```python
from build123d import *

# Parameters (mm, degrees)
SKETCH1_R                    = 6.35
EXTRUDE1_DEPTH               = 22.225
F_5_16_18_TAPPED_HOLE1_D     = 6.5278
F_5_16_18_TAPPED_HOLE1_DEPTH = 20.32
F_5_16_18_TAPPED_HOLE1_TIP   = 1.961148974
F_5_16_18_TAPPED_HOLE2_D     = 6.5278
F_5_16_18_TAPPED_HOLE2_DEPTH = 20.32
F_5_16_18_TAPPED_HOLE2_TIP   = 1.961148974
SKETCH6_W                    = 0.9906
SKETCH6_H                    = 0.4064


with BuildPart() as part:
    # Sketch1 → Extrude1 (new body, symmetric)
    with BuildSketch(Plane.XY):
        Circle(SKETCH1_R)
    extrude(amount=EXTRUDE1_DEPTH, both=True)

    # 5/16-18 Tapped Hole1
    with Locations(Plane.XY.offset(22.225)):
        with Locations((0, 0)):
            Hole(F_5_16_18_TAPPED_HOLE1_D / 2, depth=F_5_16_18_TAPPED_HOLE1_DEPTH)
            with Locations((0, 0, -(F_5_16_18_TAPPED_HOLE1_DEPTH + F_5_16_18_TAPPED_HOLE1_TIP / 2))):  # 118° drill point
                Cone(0, F_5_16_18_TAPPED_HOLE1_D / 2, F_5_16_18_TAPPED_HOLE1_TIP, mode=Mode.SUBTRACT)

    # 5/16-18 Tapped Hole2
    with Locations(Plane(origin=(0, 0, -22.225), x_dir=(-1, 0, 0), z_dir=(0, 0, -1))):
        with Locations((0, 0)):
            Hole(F_5_16_18_TAPPED_HOLE2_D / 2, depth=F_5_16_18_TAPPED_HOLE2_DEPTH)
            with Locations((0, 0, -(F_5_16_18_TAPPED_HOLE2_DEPTH + F_5_16_18_TAPPED_HOLE2_TIP / 2))):  # 118° drill point
                Cone(0, F_5_16_18_TAPPED_HOLE2_D / 2, F_5_16_18_TAPPED_HOLE2_TIP, mode=Mode.SUBTRACT)

    # Sketch6 → Cut-Revolve1 (revolve, cut)
    with BuildSketch(Plane(origin=(0, 0, 0), x_dir=(0, 0, -1), z_dir=(1, 0, 0))):
        with Locations((11.7221, 6.1468)):
            Rectangle(SKETCH6_W, SKETCH6_H)
    cut_revolve1 = revolve(axis=Axis((0, 0, 22.225), (0, 0, -1)), mode=Mode.SUBTRACT)

    # Mirror1: Cut-Revolve1 across plane
    add(cut_revolve1.mirror(Plane.XY), mode=Mode.SUBTRACT)


solid = part.part
```
Part model, mm, in its own coordinate system. A direction names the side the tool comes from. Coordinates: 2 decimals unless noted, no trailing zeros. Order: outer loops, then holes, each group sorted by start corner. A loop starts at its lowest first (then second) coordinate and runs counter-clockwise, first axis right, second up. Notation, with made-up numbers: (0.5, 61.5) -> (11.5, 61.5) arc R23 cw to (11.5, 91.5) -> close; hole circle Ø9 at (-20.5, 34). An arc over 180 degrees is marked (long way). Put each result on its own line as item: value. Start each with the question number.
(1) Mould opens along Y. For faces 4 (the face through (1.785, 5.669, 11.729)), 5 (the face through (-3, 2, 22.225)), 6 (the face through (0.708, -3.186, 11.923)) say: pulls with the +Y half, pulls with the -Y half, needs draft (parallel to the pull), parting line crosses it, or undercut.
(2) Band-saw the part on C-C (y = 5.5). Give the cut face in (x, z) (3 decimals), then the cut area to 3 significant figures.
(3) Probe line 1 along Z through (x, y) = (-4.25, -4.5) (3 decimals); line 2 along X through (y, z) = (0, 15.5). List the from-to ranges inside material, lowest first. Write a range as [from, to].
(4) Band-saw the part on B-B (x = -4). Give the cut face in (y, z) (3 decimals), then the cut area to 3 significant figures.
(5) Pin check, flat tips, straight feed: pin 1 Ø1.5 at (x, z) = (1, -14.5) entering from -Y; pin 2 Ø4 at (x, y) = (0, 0) entering from -Z. Stop position of each tip, or through.
(6) Which spindle directions (+Z, -Z, +X, -X, +Y, -Y) get a long thin tool onto all of the face, cutting with end or side? Do faces 1 (the face through (-3, 2, -22.225)), 2 (the face through (-0.708, -3.186, -11.923)), 3 (the face through (1.785, 5.669, -11.729)). Say none if no direction does.
(7) Band-saw the part on A-A (z = 15.5). Give the cut face in (x, y).
Determined:
1. face 4: parting line crosses it
1. face 5: needs draft
1. face 6: undercut
2. outline: (-3.174, -22.225) -> (3.174, -22.225) -> (3.174, -12.217) -> (2.253, -12.217) -> (2.253, -11.227) -> (3.174, -11.227) -> (3.174, 11.227) -> (2.253, 11.227) -> (2.253, 12.217) -> (3.174, 12.217) -> (3.174, 22.225) -> (-3.174, 22.225) -> (-3.174, 12.217) -> (-2.253, 12.217) -> (-2.253, 11.227) -> (-3.174, 11.227) -> (-3.174, -11.227) -> (-2.253, -11.227) -> (-2.253, -12.217) -> (-3.174, -12.217) -> close
2. area: 278 mm²
3. line 1: z = [-22.225, -12.217], [-11.227, 11.227], [12.217, 22.225]
3. line 2: x = [-6.35, -3.26], [3.26, 6.35]
4. outline: (-4.932, -22.225) -> (4.932, -22.225) -> (4.932, -12.217) -> (4.396, -12.217) -> (4.396, -11.227) -> (4.932, -11.227) -> (4.932, 11.227) -> (4.396, 11.227) -> (4.396, 12.217) -> (4.932, 12.217) -> (4.932, 22.225) -> (-4.932, 22.225) -> (-4.932, 12.217) -> (-4.396, 12.217) -> (-4.396, 11.227) -> (-4.932, 11.227) -> (-4.932, -11.227) -> (-4.396, -11.227) -> (-4.396, -12.217) -> (-4.932, -12.217) -> close
4. area: 436 mm²
5. pin 1: stops at y = -6.35
5. pin 2: stops at z = -1.15
6. face 1: -Z, +X, -X, +Y, -Y
6. face 2: -Z
6. face 3: none
7. outline: circle Ø12.7 at (0, 0); hole circle Ø6.53 at (0, 0)
